Check sheet for the drawn part. Datum: minimum x, y, z corner. Units: mm. A direction names the side the tool comes from. Coordinates: 2 decimals unless noted, no trailing zeros. Write each loop counter-clockwise with the first axis right and the second up, starting at its lowest first coordinate (ties: lowest second). Pieces come first, ordered by that corner, then holes. Notation, with made-up numbers: (-6, 78) -> (0, 78) arc R32 ccw to (0, 112) -> close; hole circle Ø2 at (61, 27.5). An arc over 180 degrees is marked (long way). Write item = value, one per line. Start each with the question number.
(1) Section check A-A (x = 27.5). Record the cut outline in (y, z), plus the area to 3 significant figures.
(2) Material ranges on probe 1 along X at (y, z) = (29, 6.75); probe 2 along Z at (x, y) = (82, 43.5); probe 3 along Y at (x, z) = (43.5, 8), recorded low to high. Write a range as [from, to].
(3) Mould release check, pull along Y, two halves, no side actions. Record for the marked faces 1, 2, 3 and 4: released by +Y, released by -Y, zero draft, split by the parting line, or undercut.
(4) Section check D-D (y = 19.5). Record the cut outline in (x, z), plus the area to 3 significant figures.
(5) Set-up check for the marked faces 5 and 6: record each of +Z, -Z, +X, -X, +Y, -Y from which the full face is reachable in a straight line by a thin tool's end or side.
(6) Gauge pin test, flat ends, axial feed: pin 1 Ø2 at (y, z) = (49.5, 2.5) entering from +X; pin 2 Ø2.5 at (y, z) = (55, 3) entering from +X; pin 3 Ø0.9 at (y, z) = (54.5, 8.5) entering from -X. Record the tip position at first contact, or that the pin passes through.
(7) Section check C-C (z = 5.5). State how many separate pieces and enclosed holes the cut face has, plus the area to 3 significant figures.
(8) Section check B-B (y = 6.5). Record the cut outline in (x, z).
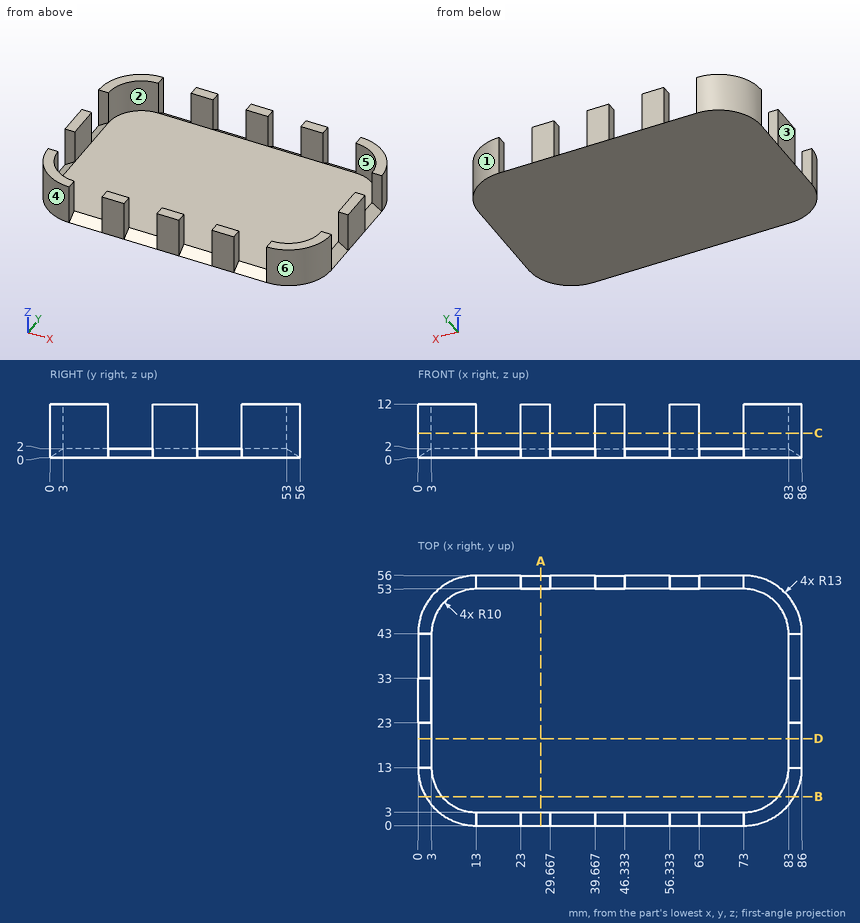
Response:
q1.outline = (0, 0) -> (56, 0) -> (56, 12) -> (53, 12) -> (53, 2) -> (3, 2) -> (3, 12) -> (0, 12) -> close
q1.area = 172 mm2
q2.probe_1 = [0, 3], [83, 86]
q2.probe_2 = [0, 2]
q2.probe_3 = [0, 3], [53, 56]
q3.face_1 = released by +Y
q3.face_2 = undercut
q3.face_3 = zero draft
q3.face_4 = released by -Y
q4.outline = (0, 0) -> (86, 0) -> (83, 2) -> (3, 2) -> close
q4.area = 166 mm2
q5.face_5 = +Z
q5.face_6 = +Z, -Z, +X, -Y
q6.pin_1 = 84.78
q6.pin_2 = 80.31
q6.pin_3 = 6.15
q7.separate_pieces = 12
q7.enclosed_holes = 0
q7.area = 397 mm2
q8.outline = (1.74, 0) -> (84.26, 0) -> (84.26, 12) -> (80.6, 12) -> (80.6, 2) -> (5.4, 2) -> (5.4, 12) -> (1.74, 12) -> close
